Could you check a few things on this model? Use its own coordinates, in mm. A direction names the side the tool comes from. Give positions to 0.01 mm unless a question says otherwise; leave off trailing zeros. Loops run counter-clockwise (first coordinate to the right, second up) from the corner with the lowest first, then second, coordinate; pieces in that order, holes last. Notation, with made-up numbers: (52, 40.5) - (76, 40.5) arc R29 cw to (76, 62.5) - close; hole circle Ø4 at (67.25, 68). An arc over 180 degrees is marked (long way). Write each question's results on one line, items separated by ' | '. Start each with the question number.
```python
from build123d import *

# Parameters (mm, degrees)
F1_DEPTH = 100
F3_DEPTH = 20
F5_DEPTH = 3
F6_R     = 2
F7_R     = 1


with BuildPart() as f1:
    # F0 (on Front) → F1 (new body)
    with BuildSketch(Plane.XZ):
        with BuildLine():
            ThreePointArc((15, 0), (0, 15), (-15, 0))
            Line((-15, 0), (-11, 0))
            Line((-11, 0), (-11, 3.297717))
            Line((-11, 3.297717), (0, 11))
            Line((0, 11), (11, 3.297717))
            Line((11, 3.297717), (11, 0))
            Line((11, 0), (15, 0))
        make_face()
    extrude(amount=F1_DEPTH)

    # F2 (on Right) → F3 (join, symmetric)
    with BuildSketch(Plane.YZ):
        Polygon((0, 20), (0, 0), (4, 0), (4, 16), (13, 16), (13, 12), (17, 12), (17, 20), align=None)
    extrude(amount=F3_DEPTH, both=True)

    # F4 (on face) → F5 (join)
    with BuildSketch(Plane.XZ.offset(100)):
        with BuildLine():
            ThreePointArc((17, 0), (0, 17), (-17, 0))
            Line((-17, 0), (17, 0))
        make_face()
    extrude(amount=F5_DEPTH)

    # F6
    f6_edges = [f1.edges().sort_by_distance(p)[0] for p in [
        (0, 17, 20),
        (0, 0, 20),
        (20, 8.5, 20),
        (-20, 8.5, 20),
        (0, 17, 12),
        (20, 0, 10),
        (-20, 0, 10),
        (-20, 17, 16),
        (20, 17, 16),
        (0, -103, 17),
    ]]
    fillet(f6_edges, radius=F6_R)

    # F7
    f7_edges = [f1.edges().sort_by_distance(p)[0] for p in [
        (0, 0, 15),
        (0, -100, 15),
    ]]
    fillet(f7_edges, radius=F7_R)


solid = f1.part
```
Q1. If we mould it in two halves opening along X, with no side actions, what happens to faces 1 (the face through (0, 9, 20)), 2 (the face through (-19.4, 0.57, 8.87)), 3 (the face through (-11, -49, 2))? For each: +X half, -X half, draft (parallel to the pull), parting line (faces both ways), or undercut.
Q2. Which directions (+Z, -Z, +X, -X, +Y, -Y) give clear straight access to the entire face, cutting with the end or side of a thin tool? Please do faces 4 (the face through (0, 13, 14)), 5 (the face through (0, -49, 15)), 6 (the face through (-5.577, -49.3, 7.095)).
Q3. I'm going to push flat-ended pins straight in: pin 1 Ø3.5 at (y, z) = (-44, 2) entering from +X; pin 2 Ø1.2 at (x, z) = (-8, 14.5) entering from -Y; pin 3 Ø5 at (y, z) = (-57.5, 11) entering from +X. Where does each tip first touch, or does it pass through?
Q4. I want a section at A-A, the plane y = -62. List the corners of the cut face in (x, z) for me, then the cut area to 3 significant figures.
Q5. I need wall thicknesses on L1, parallel to Y at x = 6, z = 3.75; L2, parallel to Y at x = -9.5, z = 13.5; L3, parallel to Y at x = -8, z = 10. Which ranges of each line are inside material? Lowest first, please. Write a range as from..to.
Conclusion:
1) face 1: draft | face 2: -X half | face 3: undercut
2) face 4: -Z, +X, -X | face 5: +Z | face 6: -Z
3) pin 1: x = 15 | pin 2: y = -102.75 | pin 3: x = 12.36
4) outline: (-15, 0) - (-11, 0) - (-11, 3.3) - (0, 11) - (11, 3.3) - (11, 0) - (15, 0) arc R15 ccw to start | area: 196 mm^2
5) L1: -103..-100, 0..4 | L2: -102.31..-100, 0..4, 13..16.94 | L3: -103..4
